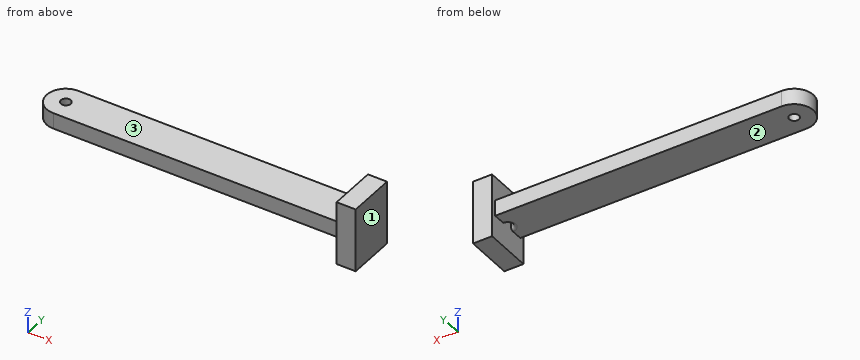
from build123d import *

# Parameters (mm, degrees)
SKETCH1_R           = 1.55
SKETCH1_R_2         = 1.5
BOSS_EXTRUDE1_DEPTH = 5
FILLET3_R           = 1
BOSS_EXTRUDE2_START = 7.5
SKETCH4_W           = 6
SKETCH4_H           = 15
BOSS_EXTRUDE2_DEPTH = 20


with BuildPart() as part:
    # Sketch1 → Boss-Extrude1 (new body)
    with BuildSketch(Plane.XY):
        with BuildLine():
            ThreePointArc((0, 6), (-6, 0), (0, -6))
            Line((0, -6), (90, -6))
            ThreePointArc((90, -6), (96, 0), (90, 6))
            Line((90, 6), (0, 6))
        make_face()
        Circle(SKETCH1_R, mode=Mode.SUBTRACT)
        with Locations((90, 0)):
            Circle(SKETCH1_R_2, mode=Mode.SUBTRACT)
    extrude(amount=BOSS_EXTRUDE1_DEPTH)

    # Fillet3
    fillet3_edges = [part.edges().sort_by_distance(p)[0] for p in [
        (88.5, 0, 0),
    ]]
    fillet(fillet3_edges, radius=FILLET3_R)

    # Sketch4 → Boss-Extrude2 (add)
    with BuildSketch(Plane.XY.offset(5).offset(BOSS_EXTRUDE2_START)):
        with Locations((93, 0)):
            Rectangle(SKETCH4_W, SKETCH4_H)
    extrude(amount=-BOSS_EXTRUDE2_DEPTH)


solid = part.part
Can you work these out from the model? Positions are in its coordinate system, mm. Face numbers are marked on the shaded views. A direction names the side the tool comes from. Coordinates: 2 decimals unless noted, no trailing zeros. Write each loop counter-clockwise with the first axis right and the second up, starting at its lowest first coordinate (ties: lowest second). Pieces come first, ordered by that corner, then holes. Notation, with made-up numbers: M 50,48 L 65,48 A29 cw 65,85 Z; hole C 53.5,66 d4. An arc over 180 degrees is marked long. Use one line per item in the form item = value.
Q1. I need wall thicknesses on line 1 along Z through (x, y) = (83, -0.75); line 2 along X through (y, z) = (2.75, 7.25); line 3 along Y through (x, z) = (14, 1). Which ranges of each line are inside material? Lowest first, please. Write a range as from..to.
Model answer:
line_1 = 0..5
line_2 = 90..96
line_3 = -6..6
Q2. If we section it at A-A (y = 0): Write out the boundary of the cut face in (x, z).
Model answer:
outline = M -6,0 L -1.55,0 L -1.55,5 L -6,5 Z; M 1.55,0 L 87.5,0 A1 ccw 88.5,1 L 88.5,5 L 1.55,5 Z; M 90,-7.5 L 96,-7.5 L 96,12.5 L 90,12.5 Z
Q3. For P1, Ø2, axis at x = 46, y = -0.5, coming from the -Z side; P2, Ø4, axis at x = 31.5, z = 2.5, coming from the -Y side; P3, Ø6, axis at x = 23.5, y = 1.5, coming from the +Z side, each with a flat end and sliding along its axis, tell me the tip position at first contact or that it passes through.
Model answer:
P1 = 0
P2 = -6
P3 = 5
Q4. If we section it at D-D (z = 10.25): Write out the boundary of the cut face in (x, y), then the cut area to 3 significant figures.
Model answer:
outline = M 90,-7.5 L 96,-7.5 L 96,7.5 L 90,7.5 Z
area = 90.0 mm^2
Q5. If we section it at B-B (x = 12.5): Write out the boundary of the cut face in (y, z).
Model answer:
outline = M -6,0 L 6,0 L 6,5 L -6,5 Z
Q6. For the marked faces 1, 2 and 3, which set-ups out of +Z, -Z, +X, -X, +Y, -Y let a thin tool reach every point of the face, with its end or its side?
Model answer:
face_1 = +Z, -Z, +X, +Y, -Y
face_2 = -Z, -X, +Y, -Y
face_3 = +Z, -X, +Y, -Y
Q7. If we section it at C-C (y = 4.75): Write out the boundary of the cut face in (x, z).
Model answer:
outline = M -3.67,0 L 90,0 L 90,-7.5 L 96,-7.5 L 96,12.5 L 90,12.5 L 90,5 L -3.67,5 Z
